The listing builds one solid part. Answer for the finished solid, in the listing's coordinates (mm). Give positions to 0.01 mm unless a question says otherwise; leave off trailing zeros. Loops run counter-clockwise (first coordinate to the right, second up) from the corner with the lowest first, then second, coordinate; pieces in that order, holes last. Notation, with made-up numbers: M -13.75,54 L 26.25,54 A30 cw 26.25,88 Z; hole C 10,66.5 d11. An arc over 180 degrees is marked long. One line per item, written item: value. Start each with the question number.
Q1. Consider L1, parallel to Z at x = -54.5, y = 2.45; L2, parallel to Z at x = -53, y = 1.95; L3, parallel to X at y = 3.2, z = -28.5. Determine where each line is inside the solid, lowest interval first.
Q2. A cutting plane is placed at A-A, the plane x = -56.5. Determine the outline of the cut face in (y, z) (3 decimals), and give its area (3 significant figures).
Q3. Flat-ended cylindrical pins translate along their axes: pin 1 (3.5 mm diameter, centred on x = -54.88, z = -25.91, fed in from -Y); pin 2 (10 mm diameter, centred on x = -34.5, z = -62.5, fed in from -Y). Find the tip coordinate at first contact, or state that the pin passes through.
Autodesk Inventor part; units mm, degrees
ref_plane "YZ Plane" through (0, 0, 0) normal (1, 0, 0) x (0, 1, 0)
ref_plane "XZ Plane" through (0, 0, 0) normal (0, 1, 0) x (-1, 0, 0)
ref_plane "XY Plane" through (0, 0, 0) normal (0, 0, 1) x (1, 0, 0)
sketch "Sketch1" plane through (0, 0, 0) normal (0, 1, 0) x (-1, 0, 0)
  line L0 (0, 0) -> (0, -120)
  line L1 (0, -120) -> (70, -120)
  line L2 (70, -120) -> (70, 0)
  line L3 (70, 0) -> (0, 0)
  line L4 (70, 0) -> (0, 0)
  dimension "d0" = 120
  dimension "d1" = 70
extrude "Extrusion1" add sketch "Sketch1" along normal blind 5.5
sketch "Sketch2" plane through (0, 5.5, 0) normal (0, 1, 0) x (1, 0, 0)
  line L0 (0, 120) -> (-70, 120) construction
  line L1 (0, 0) -> (0, 120) construction
  line L2 (-70, 120) -> (0, 0) construction
  line L3 (-70, 0) -> (0, 0) construction
  line L4 (-70, 0) -> (0, 120) construction
  line L5 (-70, 120) -> (-54.8839, 94.0866) construction
  line L6 (-70, 0) -> (-54.8839, 25.9134) construction
  dimension "d4" = 30
  dimension "d5" = 30
hole "Hole1" at (-54.8839, 5.5, -94.0866) at (-54.8839, 5.5, -25.9134) direction (0, -1, 0) diameter 5.9175 depth 19.1 tip angle 118
properties part number "HL"
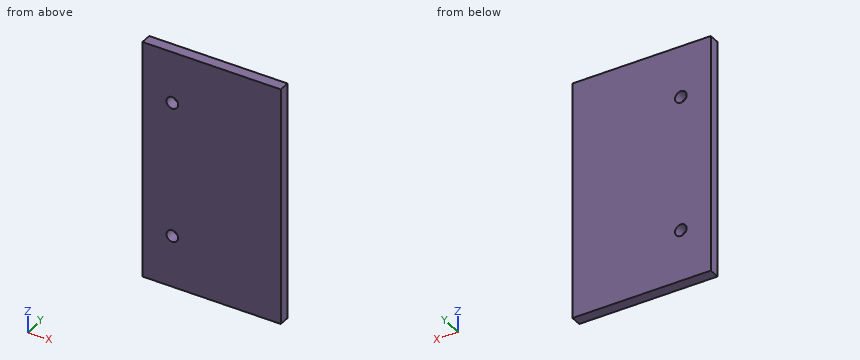
Answer block:
1. L1: -120 to -97.02, -91.15 to -28.85, -22.98 to 0
1. L2: -120 to -96.37, -91.81 to -28.19, -23.63 to 0
1. L3: -70 to -56.32, -53.45 to 0
2. outline: M 0,-120 L 5.5,-120 L 5.5,-96.565 L 0,-96.565 Z; M 0,-91.608 L 5.5,-91.608 L 5.5,-28.392 L 0,-28.392 Z; M 0,-23.435 L 5.5,-23.435 L 5.5,0 L 0,0 Z
2. area: 605 mm^2
3. pin 1: through
3. pin 2: y = 0
